Geometry: final body of the model. Coordinates: model frame, mm. A direction names the side the tool comes from. Coordinates: 2 decimals unless noted, no trailing zeros. Order: outer loops, then holes, each group sorted by start corner. A loop starts at its lowest first (then second) coordinate and runs counter-clockwise, first axis right, second up. Notation, with made-up numbers: M 44,3.5 L 102,3.5 A16 ccw 102,11.5 Z; hole C -15,-7 d10. An arc over 180 degrees is marked long. Use CSV: the item, a comma, the result in double quotes. Start each with the question number.
Q1. Access query for faces 5 (the face through (41.81, -47, 2)), 6 (the face through (37.81, 15, 3)), 7 (the face through (30.81, 10, 1)), 8 (the face through (43, -34, 3)). Directions: +Z, -Z, +X, -X, +Y, -Y. A direction counts if a zero-diameter tool reaches every point of the face in a straight line with its end or side. Return the directions, or none.
Q2. Section query C-C, the plane y = 2.5. Output: boundary loops of the cut face in (x, z), and give its area (3 significant figures).
Q3. Section query A-A, the plane z = 2.75. Output: boundary loops of the cut face in (x, y).
Q4. First-contact query: P1, Ø12, axis at x = -24.5, y = -35, coming from the +Z side; P2, Ø3, axis at x = 30, z = 1, coming from the -Y side. Flat tips, straight axial feed; report the tip coordinate or a pass-through.
Q5. Mould query, pull axis X, two halves, no side actions, for faces 1 (the face through (2, 0, 1)), 2 (the face through (-38.94, -47, 2)), 3 (the face through (43, 15, 5)), 4 (the face through (-44.94, -15, 1)). Classes: +X half, -X half, draft (parallel to the pull), parting line (faces both ways), or undercut.
Q6. Ray query, probe 1 along X at (y, z) = (-47.4, 3.15); probe 2 along X at (y, z) = (8, 1.9); probe 3 along X at (y, z) = (11, 4.7). Return the intervals inside material, ascending.
Q7. Section query B-B, the plane y = -47.4. Output: boundary loops of the cut face in (x, z).
Q8. Section query D-D, the plane y = 17.6. Output: boundary loops of the cut face in (x, z).
from build123d import *

# Parameters (mm, degrees)
F0_R     = 1.6
F1_DEPTH = 2
F2_W     = 10
F2_H     = 10
F2_R     = 1.6
F3_DEPTH = 3
F4_W     = 6
F4_H     = 6
F4_R     = 1.6
F5_DEPTH = 5


with BuildPart() as f1:
    # F0 (on Top) → F1 (new body)
    with BuildSketch(Plane.XY):
        Polygon((-27.939597, 0), (-27.939597, 20), (-44.939597, 20), (-44.939597, -44), (47.810403, -44), (47.810403, 20), (30.810403, 20), (30.810403, 0), align=None)
        with Locations((-42.539597, 17.6)):
            Circle(F0_R, mode=Mode.SUBTRACT)
        with Locations((45.410403, 17.6)):
            Circle(F0_R, mode=Mode.SUBTRACT)
    extrude(amount=F1_DEPTH)

    # F2 (on face) → F3 (join)
    with BuildSketch(Plane.XY.offset(2)):
        with Locations((-39.939597, 15)):
            Rectangle(F2_W, F2_H)
        with Locations((-42.539597, 17.6)):
            Circle(F2_R, mode=Mode.SUBTRACT)
        with Locations((42.810403, 15)):
            Rectangle(F2_W, F2_H)
        with Locations((45.410403, 17.6)):
            Circle(F2_R, mode=Mode.SUBTRACT)
        with Locations((-39.939597, -39)):
            Rectangle(F2_W, F2_H)
        with Locations((42.810403, -39)):
            Rectangle(F2_W, F2_H)
    extrude(amount=F3_DEPTH)

    # F4 (on face) → F5 (join)
    with BuildSketch(Plane(origin=(0, 0, 0), x_dir=(1, 0, 0), z_dir=(0, 0, -1))):
        with Locations((-41.939597, 47)):
            Rectangle(F4_W, F4_H)
        with Locations((-42.539597, 47.4)):
            Circle(F4_R, mode=Mode.SUBTRACT)
        with Locations((44.810403, 47)):
            Rectangle(F4_W, F4_H)
        with Locations((45.410403, 47.4)):
            Circle(F4_R, mode=Mode.SUBTRACT)
    extrude(amount=-F5_DEPTH)


solid = f1.part
Responses:
1,face 5,"+Z, -Z, -Y"
1,face 6,"+Z, +Y, -Y"
1,face 7,"+Z, -Z, +Y"
1,face 8,"+Z, +X, -X"
2,outline,"M -44.94,0 L -27.94,0 L -27.94,2 L -44.94,2 Z; M 30.81,0 L 47.81,0 L 47.81,2 L 30.81,2 Z"
2,area,"68.0 mm²"
3,outline,"M -44.94,-50 L -38.94,-50 L -38.94,-44 L -34.94,-44 L -34.94,-34 L -44.94,-34 Z; M -44.94,10 L -34.94,10 L -34.94,20 L -44.94,20 Z; M 37.81,-44 L 41.81,-44 L 41.81,-50 L 47.81,-50 L 47.81,-34 L 37.81,-34 Z; M 37.81,10 L 47.81,10 L 47.81,20 L 37.81,20 Z; hole C -42.54,-47.4 d3.2; hole C -42.54,17.6 d3.2; hole C 45.41,-47.4 d3.2; hole C 45.41,17.6 d3.2"
4,P1,"stops at z = 2"
4,P2,"stops at y = -44"
5,face 1,"undercut"
5,face 2,"undercut"
5,face 3,"draft"
5,face 4,"-X half"
6,probe 1,"x = -44.94 to -44.14, -40.94 to -38.94, 41.81 to 43.81, 47.01 to 47.81"
6,probe 2,"x = -44.94 to -27.94, 30.81 to 47.81"
6,probe 3,"x = -44.94 to -34.94, 37.81 to 47.81"
7,outline,"M -44.94,0 L -44.14,0 L -44.14,5 L -44.94,5 Z; M -40.94,0 L -38.94,0 L -38.94,5 L -40.94,5 Z; M 41.81,0 L 43.81,0 L 43.81,5 L 41.81,5 Z; M 47.01,0 L 47.81,0 L 47.81,5 L 47.01,5 Z"
8,outline,"M -44.94,0 L -44.14,0 L -44.14,5 L -44.94,5 Z; M -40.94,0 L -27.94,0 L -27.94,2 L -34.94,2 L -34.94,5 L -40.94,5 Z; M 30.81,0 L 43.81,0 L 43.81,5 L 37.81,5 L 37.81,2 L 30.81,2 Z; M 47.01,0 L 47.81,0 L 47.81,5 L 47.01,5 Z"
